Autodesk Inventor part; units mm, degrees
ref_plane "YZ Plane" through (0, 0, 0) normal (1, 0, 0) x (0, 1, 0)
ref_plane "XZ Plane" through (0, 0, 0) normal (0, 1, 0) x (-1, 0, 0)
ref_plane "XY Plane" through (0, 0, 0) normal (0, 0, 1) x (1, 0, 0)
sketch "Sketch1" plane through (0, 0, 0) normal (0, 1, 0) x (-1, 0, 0)
  line L0 (0, 0) -> (-440, 0)
  line L1 (-440, 0) -> (-440, -440)
  line L2 (-440, -440) -> (0, -440)
  line L3 (0, -440) -> (0, 0)
  line L4 (-76.8377, -361.5) -> (-76.8377, -358.5)
  arc A0 (-76.8377, -358.5) -> (-76.8377, -361.5) centre (-80, -360) ccw
  line L5 (-156.8377, -361.5) -> (-156.8377, -358.5)
  arc A1 (-156.8377, -358.5) -> (-156.8377, -361.5) centre (-160, -360) ccw
  line L6 (-76.8377, -301.5) -> (-76.8377, -298.5)
  arc A2 (-76.8377, -298.5) -> (-76.8377, -301.5) centre (-80, -300) ccw
  line L7 (-156.8377, -301.5) -> (-156.8377, -298.5)
  arc A3 (-156.8377, -298.5) -> (-156.8377, -301.5) centre (-160, -300) ccw
  line L8 (-76.8377, -241.5) -> (-76.8377, -238.5)
  arc A4 (-76.8377, -238.5) -> (-76.8377, -241.5) centre (-80, -240) ccw
  line L9 (-156.8377, -241.5) -> (-156.8377, -238.5)
  arc A5 (-156.8377, -238.5) -> (-156.8377, -241.5) centre (-160, -240) ccw
  line L10 (-76.8377, -181.5) -> (-76.8377, -178.5)
  arc A6 (-76.8377, -178.5) -> (-76.8377, -181.5) centre (-80, -180) ccw
  line L11 (-156.8377, -181.5) -> (-156.8377, -178.5)
  arc A7 (-156.8377, -178.5) -> (-156.8377, -181.5) centre (-160, -180) ccw
  line L12 (-76.8377, -121.5) -> (-76.8377, -118.5)
  arc A8 (-76.8377, -118.5) -> (-76.8377, -121.5) centre (-80, -120) ccw
  line L13 (-156.8377, -121.5) -> (-156.8377, -118.5)
  arc A9 (-156.8377, -118.5) -> (-156.8377, -121.5) centre (-160, -120) ccw
  line L14 (-76.8377, -61.5) -> (-76.8377, -58.5)
  arc A10 (-76.8377, -58.5) -> (-76.8377, -61.5) centre (-80, -60) ccw
  line L15 (-156.8377, -61.5) -> (-156.8377, -58.5)
  arc A11 (-156.8377, -58.5) -> (-156.8377, -61.5) centre (-160, -60) ccw
  circle A12 centre (-340, -360) radius 14
  circle A13 centre (-340, -360) radius 17.5 construction
  line L16 (-340, -360) -> (-390.216, -360) construction
  line L17 (-340, -360) -> (-300.4396, -360) construction
  line L18 (-340, -360) -> (-352.3744, -372.3744) construction
  line L19 (-340, -360) -> (-327.6256, -372.3744) construction
  line L20 (-340, -360) -> (-327.6256, -347.6256) construction
  line L21 (-340, -360) -> (-353.5956, -346.4044) construction
  circle A14 centre (-352.3744, -347.6256) radius 2
  circle A15 centre (-327.6256, -347.6256) radius 2
  circle A16 centre (-327.6256, -372.3744) radius 2
  circle A17 centre (-352.3744, -372.3744) radius 2
  circle A18 centre (-327.6256, -252.3744) radius 2
  circle A19 centre (-352.3744, -252.3744) radius 2
  circle A20 centre (-340, -240) radius 14
  circle A21 centre (-327.6256, -227.6256) radius 2
  circle A22 centre (-352.3744, -227.6256) radius 2
  circle A23 centre (-327.6256, -132.3744) radius 2
  circle A24 centre (-352.3744, -132.3744) radius 2
  circle A25 centre (-340, -120) radius 14
  circle A26 centre (-327.6256, -107.6256) radius 2
  circle A27 centre (-352.3744, -107.6256) radius 2
  circle A28 centre (-240, -300) radius 14
  circle A29 centre (-240, -300) radius 17.5 construction
  line L22 (-240, -300) -> (-290.216, -300) construction
  line L23 (-240, -300) -> (-200.4396, -300) construction
  line L24 (-240, -300) -> (-252.3744, -312.3744) construction
  line L25 (-240, -300) -> (-227.6256, -312.3744) construction
  line L26 (-240, -300) -> (-227.6256, -287.6256) construction
  line L27 (-240, -300) -> (-253.5956, -286.4044) construction
  circle A30 centre (-252.3744, -287.6256) radius 2
  circle A31 centre (-227.6256, -287.6256) radius 2
  circle A32 centre (-227.6256, -312.3744) radius 2
  circle A33 centre (-252.3744, -312.3744) radius 2
  line L28 (-240, -180) -> (-290.216, -180) construction
  circle A34 centre (-252.3744, -192.3744) radius 2
  line L29 (-240, -180) -> (-252.3744, -192.3744) construction
  circle A35 centre (-252.3744, -167.6256) radius 2
  line L30 (-240, -180) -> (-253.5956, -166.4044) construction
  line L31 (-240, -180) -> (-227.6256, -192.3744) construction
  circle A36 centre (-227.6256, -192.3744) radius 2
  line L32 (-240, -180) -> (-227.6256, -167.6256) construction
  circle A37 centre (-240, -180) radius 14
  circle A38 centre (-240, -180) radius 17.5 construction
  circle A39 centre (-227.6256, -167.6256) radius 2
  line L33 (-240, -180) -> (-200.4396, -180) construction
  line L34 (-240, -60) -> (-290.216, -60) construction
  circle A40 centre (-252.3744, -72.3744) radius 2
  line L35 (-240, -60) -> (-252.3744, -72.3744) construction
  circle A41 centre (-252.3744, -47.6256) radius 2
  line L36 (-240, -60) -> (-253.5956, -46.4044) construction
  line L37 (-240, -60) -> (-227.6256, -72.3744) construction
  circle A42 centre (-227.6256, -72.3744) radius 2
  line L38 (-240, -60) -> (-227.6256, -47.6256) construction
  circle A43 centre (-240, -60) radius 14
  circle A44 centre (-240, -60) radius 17.5 construction
  circle A45 centre (-227.6256, -47.6256) radius 2
  line L39 (-240, -60) -> (-200.4396, -60) construction
  dimension "d0" = 440
  dimension "d1" = 440
  dimension "d107" = 3.5
  dimension "d109" = 3
  dimension "d111" = 80
  dimension "d135" = 80
  dimension "d138" = 80
  dimension "d141" = 60
  dimension "d163" = 28
  dimension "d164" = 35
  dimension "d166" = 45
  dimension "d167" = 45
  dimension "d169" = 45
  dimension "d170" = 45
  dimension "d171" = 4
  dimension "d172" = 4
  dimension "d173" = 4
  dimension "d174" = 80
  dimension "d176" = 4
  dimension "d179" = 120
  dimension "d184" = 28
  dimension "d185" = 35
  dimension "d186" = 45
  dimension "d187" = 45
  dimension "d188" = 45
  dimension "d189" = 45
  dimension "d190" = 4
  dimension "d191" = 4
  dimension "d192" = 4
  dimension "d193" = 4
  dimension "d194" = 200
  dimension "d195" = 140
  dimension "d198" = 120
  dimension "d205" = 100
extrude "Extrusion5" add sketch "Sketch1" along normal blind 6
properties part number "panel"
Build history of the part. All positions in model axes, mm. Coordinates: 2 decimals unless noted, no trailing zeros. Order: outer loops, then holes, each group sorted by start corner. A loop starts at its lowest first (then second) coordinate and runs counter-clockwise, first axis right, second up.
Item 1: Saw through at A-A on x = 240. List the corners of the cut face in (y, z).
Filled in:
outline: (0, -440) - (6, -440) - (6, -314) - (0, -314) - close; (0, -286) - (6, -286) - (6, -194) - (0, -194) - close; (0, -166) - (6, -166) - (6, -74) - (0, -74) - close; (0, -46) - (6, -46) - (6, 0) - (0, 0) - close
Item 2: Saw through at B-B on y = 4.5. State how many separate pieces and enclosed holes the cut face has, then the cut area to 3 significant figures.
Filled in:
separate pieces: 1
enclosed holes: 42
area: 189,000 mm2
Item 3: Drill centre lines: L1, parallel to Z at x = 340, y = 1.8; L2, parallel to X at y = 3, z = -168; L3, parallel to Z at x = 332, y = 4.3. Where is each one in solid material? Low to high.
Filled in:
L1: z = -440 to -374, -346 to -254, -226 to -134, -106 to 0
L2: x = 0 to 225.66, 229.59 to 232.79, 247.21 to 250.41, 254.34 to 440
L3: z = -440 to -371.49, -348.51 to -251.49, -228.51 to -131.49, -108.51 to 0
Item 4: Mould opens along X. For faces 1 (the flat face through (223, 6, -217)), 2 (the cylindrical face through (333.5, 3, -347.6)), 3 (the cylindrical face through (327.068, 2.958, -234.638)) say: released by +X, released by -X, zero draft, split by the parting line, or undercut.
Filled in:
face 1: zero draft
face 2: undercut
face 3: undercut
